Work out the finished part from the listing and answer in its coordinate system (mm). Face numbers are marked on the shaded views. A direction names the side the tool comes from. Give positions to 0.01 mm unless a question says otherwise; leave off trailing zeros. Order: outer loops, then holes, each group sorted by start corner. A loop starts at its lowest first (then second) coordinate and runs counter-clockwise, first axis right, second up.
```python
from build123d import *

# Parameters (mm, degrees)
F1_DEPTH        = 45
F2_R            = 2
F3_R            = 2.5
F5_DEPTH        = 2
F6_R            = 4
F7_DEPTH        = 23.5
F8_SIZE2        = 2.31
F8_SIZE         = 4
F10_D           = 6
F10_CSINK_D     = 9.5
F10_CSINK_ANGLE = 90
F11_R           = 6.5
F12_DEPTH       = 2
F14_W           = 5
F14_H           = 11
F15_DEPTH       = 25
F16_D           = 6
F16_CSINK_D     = 9.5
F16_CSINK_ANGLE = 90


# Not quite as in the source:
# - a fillet or chamfer that OpenCascade refuses, or shapes differently, is made with other operations: its cross-section is extruded or revolved along the edge and cut away or added
# - a feature names something its author has since deleted; it is built from what else it names


with BuildPart() as f1:
    # F0 (on Front) → F1 (new body)
    with BuildSketch(Plane.XZ):
        with BuildLine():
            Line((31.1786754111, 1.25), (6.3786754111, 1.25))
            ThreePointArc((6.3786754111, 1.25), (-6.5, 0), (6.3786754111, -1.25))
            Line((6.3786754111, -1.25), (33.6786754111, -1.25))
            Line((33.6786754111, -1.25), (33.6786754111, 5.75))
            Line((33.6786754111, 5.75), (43.1786754111, 5.75))
            Line((43.1786754111, 5.75), (43.1786754111, 8.25))
            Line((43.1786754111, 8.25), (31.1786754111, 8.25))
            Line((31.1786754111, 8.25), (31.1786754111, 1.25))
        make_face()
    extrude(amount=F1_DEPTH)

    # F2
    f2_edges = [f1.edges().sort_by_distance(p)[0] for p in [
        (43.178675, -45, 7),
        (43.178675, 0, 7),
    ]]
    fillet(f2_edges, radius=F2_R)

    # F3
    f3_edges = [f1.edges().sort_by_distance(p)[0] for p in [
        (33.678675, -22.5, -1.25),
        (31.178675, -22.5, 8.25),
    ]]
    fillet(f3_edges, radius=F3_R)

    # F4 (on face) → F5 (join)
    with BuildSketch(Plane(origin=(0, 0, 0), x_dir=(-1, 0, 0), z_dir=(0, 1, 0))):
        with BuildLine():
            ThreePointArc((-6.3786754111, -1.25), (0.6279370303, -6.469597753), (6.5, 0))
            ThreePointArc((6.5, 0), (0.6279370303, 6.469597753), (-6.3786754111, 1.25))
            ThreePointArc((-6.3786754111, 1.25), (-6.5, 0), (-6.3786754111, -1.25))
        make_face()
    extrude(amount=F5_DEPTH)

    # F6 (on face) → F7 (join)
    with BuildSketch(Plane(origin=(0, 2, 0), x_dir=(-1, 0, 0), z_dir=(0, 1, 0))):
        Circle(F6_R)
    extrude(amount=F7_DEPTH)

    # F8
    f8_edges = [f1.edges().sort_by_distance(p)[0] for p in [
        (4, 25.5, 0),
    ]]
    f8_side = f1.faces().sort_by_distance((4, 13.75, 0))[0]
    chamfer(f8_edges, length=F8_SIZE, length2=F8_SIZE2, reference=f8_side)

    # F10 (through all)
    with Locations(Plane(origin=(0, 0, -1.25), x_dir=(1, 0, 0), z_dir=(0, 0, -1))):
        with Locations((22.8786754111, 6.6), (17.8786754111, 37.8)):
            CounterSinkHole(F10_D / 2, F10_CSINK_D / 2, counter_sink_angle=F10_CSINK_ANGLE)

    # F11 (on face) → F12 (join)
    with BuildSketch(Plane.XZ.offset(45)):
        Circle(F11_R)
    extrude(amount=F12_DEPTH)

    # F13: fillet of radius 2 on 1 edges, made by hand

    # F13_s1 → F13_t2 (revolve, cut)
    with BuildSketch(Plane.XY):
        with BuildLine():
            ThreePointArc((6.5, -45), (5.9142135624, -46.4142135624), (4.5, -47))
            Line((4.5, -47), (6.5, -47))
            Line((6.5, -47), (6.5, -45))
        make_face()
    revolve(axis=Axis((0, -47, 0), (0, -1, 0)), mode=Mode.SUBTRACT)

    # F14 (on face) → F15 (cut)
    with BuildSketch(Plane(origin=(0, 0, 5.75), x_dir=(1, 0, 0), z_dir=(0, 0, -1))):
        with Locations((33.6786754111, 22.2)):
            Rectangle(F14_W, F14_H)
    extrude(amount=F15_DEPTH, mode=Mode.SUBTRACT)

    # F16 (through all)
    with Locations(Plane(origin=(0, 0, 5.75), x_dir=(1, 0, 0), z_dir=(0, 0, -1))):
        with Locations((37.6786754111, 22.2)):
            CounterSinkHole(F16_D / 2, F16_CSINK_D / 2, counter_sink_angle=F16_CSINK_ANGLE)


solid = f1.part
```
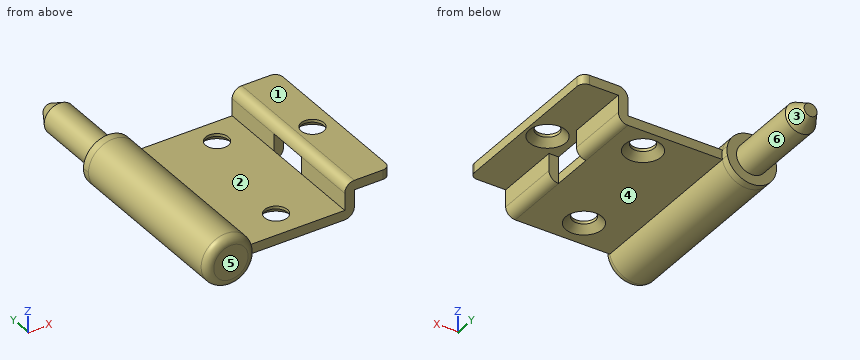
1. Which of the six approach directions +Z, -Z, +X, -X, +Y, -Y give full straight-line access (tool end or side, diameter ignored) to the marked faces 4, 5 and 6?
Findings below:
face 4: -Z, +X, +Y, -Y
face 5: +Z, -Z, +X, -X, -Y
face 6: +Y
2. Straight lines are drawn through the part: probe 1 along Y at (x, z) = (33, 5.25); probe 2 along Z at (x, y) = (7.5, -14). For each, find the intervals that lie inside material, in ascending order.
Findings below:
probe 1: y = -45 to -27.7, -16.7 to 0
probe 2: z = -1.25 to 1.25
3. Given P1, Ø2, axis at x = 6.5, y = 18, coming from the +Z side; P2, Ø5, axis at y = -37, z = 4, coming from the -X side; P3, Ø1.2, axis at x = 32, z = 1, coming from the -Y side; P4, Ø4, axis at x = 12.5, y = -27.5, coming from the +Z side, each flat-ended and moving along its own axis, determine where each tip first touches the part or whether it passes through.
Findings below:
P1: passes through
P2: stops at x = -6.32
P3: stops at y = -45
P4: stops at z = 1.25
4. The part is cut by section B-B (x = 0). Write down the section's boundary in (y, z), then the cut area to 3 significant figures.
Findings below:
outline: (-47, -4.5) arc R2 ccw to (-45, -6.5) - (2, -6.5) - (2, -4) - (21.5, -4) - (25.5, -1.69) - (25.5, 1.69) - (21.5, 4) - (2, 4) - (2, 6.5) - (-45, 6.5) arc R2 ccw to (-47, 4.5) - close
area: 814 mm2
5. The mould has two halves that part along X. Classify the marked faces 1, 2 and 3: pulls with the +X half, pulls with the -X half, needs draft (parallel to the pull), parting line crosses it, or undercut.
Findings below:
face 1: needs draft
face 2: undercut
face 3: parting line crosses it
6. The part is cut by section A-A (y = -6.6). Write down the section's boundary in (x, z).
Findings below:
outline: (6.38, -1.25) - (18.13, -1.25) - (19.88, 0.5) - (19.88, 1.25) - (6.38, 1.25) arc R6.5 ccw (long way) to start; (25.88, 0.5) - (27.63, -1.25) - (31.18, -1.25) arc R2.5 ccw to (33.68, 1.25) - (33.68, 5.75) - (43.18, 5.75) - (43.18, 8.25) - (33.68, 8.25) arc R2.5 ccw to (31.18, 5.75) - (31.18, 1.25) - (25.88, 1.25) - close
7. The part is cut by section C-C (y = -23). State how many separate pieces and enclosed holes the cut face has, then the cut area to 3 significant figures.
Findings below:
separate pieces: 3
enclosed holes: 0
area: 206 mm2
8. The part is cut by section D-D (y = 11.5). Write down the section's boundary in (x, z), then the cut area to 3 significant figures.
Findings below:
outline: circle Ø8 at (0, 0)
area: 50.3 mm2
